CAD build for the part. Positions are in the model's coordinates, mm. A direction names the side the tool comes from. Give positions to 0.01 mm unless a question says otherwise; leave off trailing zeros. Order: outer loops, then holes, each group sorted by start corner. A loop starts at its lowest first (then second) coordinate and runs counter-clockwise, first axis right, second up. Notation, with made-up numbers: M -22,84 L 19,84 A15 cw 19,102 Z; hole C 33,23.25 d4. An arc over 180 degrees is marked long. Put each result on its own line as item: value. Start each with the question number.
1) Cut at D-D (y = 0.5). Write the cut outline in (x, z), and give its area (3 significant figures).
2) Tool access for faces 1 (the face through (-5.53, 7.15, 1.97)), 2 (the face through (15.57, 2.73, 2.03)): list every direction of +Z, -Z, +X, -X, +Y, -Y with a clear straight run to the whole face (end or side of a thin tool).
3) Cut at A-A (z = 2.3). Write the cut outline in (x, y).
4) Pin check, flat tips, straight feed: pin 1 (1 mm diameter, centred on x = -6.5, z = 3, fed in from +Y); pin 2 (6.5 mm diameter, centred on x = 0, y = 0, fed in from +Z). Stop position of each tip, or through.
5) Cut at C-C (y = 13). Write the cut outline in (x, z), and give its area (3 significant figures).
6) Drill centre lines: line 1 (Y direction, x = 0, z = 1.3); line 2 (X direction, y = 9, z = 3.1); line 3 (X direction, y = 11.5, z = 2.6). Where is each one in solid material? Low to high. Write a range as [from, to].
7) Cut at B-B (x = -1.5). Write the cut outline in (y, z), and give its area (3 significant figures).
```python
from build123d import *

# Parameters (mm, degrees)
SKETCH_1_R      = 2.5
EXTRUDE_1_DEPTH = 4
FILLET_1_R      = 5


with BuildPart() as part:
    # ｽｹｯﾁ1 → ﾎﾞｽ - 押し出し1 (new body)
    with BuildSketch(Plane.XY):
        Polygon((9.00034941, 21), (-9.00034941, 21), (-15.647843116, 2.736161147), (-15.647843116, -2.584727716), (-5.344155371, -9.396926208), (5.344155371, -9.396926208), (15.647843116, -2.584727716), (15.647843116, 2.736161147), align=None)
        Circle(SKETCH_1_R, mode=Mode.SUBTRACT)
        Polygon((-11.889072633, 1.368080573), (-6.758770483, 15.463469885), (-3, 14.095389312), (-8.13030215, 0), align=None, mode=Mode.SUBTRACT)
        Polygon((8.13030215, 0), (3, 14.095389312), (6.758770483, 15.463469885), (11.889072633, 1.368080573), align=None, mode=Mode.SUBTRACT)
    extrude(amount=EXTRUDE_1_DEPTH)

    # ﾌｨﾚｯﾄ1
    fillet_1_edges = [part.edges().sort_by_distance(p)[0] for p in [
        (-15.647843116, 2.736161147, 2),
        (-9.00034941, 21, 2),
        (9.00034941, 21, 2),
        (15.647843116, 2.736161147, 2),
        (15.647843116, -2.584727716, 2),
        (5.344155371, -9.396926208, 2),
        (-5.344155371, -9.396926208, 2),
        (-15.647843116, -2.584727716, 2),
    ]]
    fillet(fillet_1_edges, radius=FILLET_1_R)


solid = part.part
```
Solution:
1. outline: M -15.65,0 L -9.5,0 L -9.5,4 L -15.65,4 Z; M -7.95,0 L -2.45,0 L -2.45,4 L -7.95,4 Z; M 2.45,0 L 7.95,0 L 7.95,4 L 2.45,4 Z; M 9.5,0 L 15.65,0 L 15.65,4 L 9.5,4 Z
1. area: 93.1 mm²
2. face 1: +Z, -Z
2. face 2: +Z, -Z, +X, +Y
3. outline: M -15.65,0.1 A5 ccw -13.41,-4.07 L -6.6,-8.57 A5 ccw -3.84,-9.4 L 3.84,-9.4 A5 ccw 6.6,-8.57 L 13.41,-4.07 A5 ccw 15.65,0.1 L 15.65,1.85 A5 ccw 15.35,3.56 L 10.2,17.71 A5 ccw 5.5,21 L -5.5,21 A5 ccw -10.2,17.71 L -15.35,3.56 A5 ccw -15.65,1.85 Z; hole M -11.89,1.37 L -8.13,0 L -3,14.1 L -6.76,15.46 Z; hole C 0,0 d5; hole M 3,14.1 L 8.13,0 L 11.89,1.37 L 6.76,15.46 Z
4. pin 1: y = 20.97
4. pin 2: z = 4
5. outline: M -11.91,0 L -7.66,0 L -7.66,4 L -11.91,4 Z; M -3.4,0 L 3.4,0 L 3.4,4 L -3.4,4 Z; M 7.66,0 L 11.91,0 L 11.91,4 L 7.66,4 Z
5. area: 61.2 mm²
6. line 1: [-9.4, -2.5], [2.5, 21]
6. line 2: [-13.37, -9.11], [-4.85, 4.85], [9.11, 13.37]
6. line 3: [-12.46, -8.2], [-3.94, 3.94], [8.2, 12.46]
7. outline: M -9.4,0 L -2,0 L -2,4 L -9.4,4 Z; M 2,0 L 21,0 L 21,4 L 2,4 Z
7. area: 106 mm²
